Here's how the part is built. I have some questions about the finished solid (model axes, mm). A direction names the side the tool comes from. Coordinates: 2 decimals unless noted, no trailing zeros. Write each loop counter-clockwise with the first axis right and the second up, starting at its lowest first coordinate (ties: lowest second). Pieces come first, ordered by that corner, then holes.
Autodesk Inventor part; units mm, degrees
ref_plane "YZ Plane" through (0, 0, 0) normal (1, 0, 0) x (0, 1, 0)
ref_plane "XZ Plane" through (0, 0, 0) normal (0, 1, 0) x (-1, 0, 0)
ref_plane "XY Plane" through (0, 0, 0) normal (0, 0, 1) x (1, 0, 0)
sketch "Esboço1" plane through (0, 0, 0) normal (0, 1, 0) x (-1, 0, 0)
  line L0 (-20.5, 23.5) -> (20.5, 23.5)
  line L1 (20.5, 23.5) -> (20.5, -23.5)
  line L2 (20.5, -23.5) -> (-20.5, -23.5)
  line L3 (-20.5, -23.5) -> (-20.5, 23.5)
  line L4 (-20.5, 23.5) -> (20.5, -23.5) construction
  line L5 (20.5, 23.5) -> (-20.5, -23.5) construction
  point P0 (0, 0)
  dimension "d0" = 41
  dimension "d1" = 47
extrude "Extrusão1" add sketch "Esboço1" along normal blind 61
shell "Casca1" thickness 2 removed faces 2 at (6.8333, 20.3333, 23.5) at (20.5, 20.3333, -7.8333)
sketch "Esboço4" plane through (-20.5, 0, 23.5) normal (0, 0, 1) x (1, 0, 0)
  line L0 (2, 2) -> (2, 59)
  line L1 (2, 59) -> (15, 59)
  line L2 (15, 59) -> (15, 54.5)
  line L3 (15, 54.5) -> (2, 54.5)
  line L4 (2, 54.5) -> (2, 59)
  line L5 (41, 2) -> (2, 2)
  line L6 (2, 2) -> (15, 2)
  line L7 (15, 2) -> (15, 7.5)
  line L8 (15, 7.5) -> (2, 7.5)
  line L9 (2, 7.5) -> (2, 2)
  arc A0 (7.6282, 59) -> (9.3718, 59) centre (8.5, 57.2) ccw
  circle A1 centre (8.3, 4.5) radius 2
  line L10 (41, 0) -> (0, 0)
  line L11 (0, 0) -> (0, 61)
  line L12 (0, 61) -> (41, 61)
  point P0 (20.5, 0)
  dimension "d15" = 13
  dimension "d16" = 4.5
  dimension "d17" = 13
  dimension "d18" = 5.5
  dimension "d19" = 4
  dimension "d20" = 4
  dimension "d21" = 4.5
  dimension "d22" = 8.3
  dimension "d23" = 3.8
  dimension "d24" = 8.5
extrude "Extrusão2" add sketch "Esboço4" against normal blind 3 contours L0 L1 A0 L2 L3 | L0 L8 L7 L5
fillet "Arredondamento4" radius 4 2 edges at (20.5, 60, 23.5) (20.5, 1, 23.5)
sketch "Esboço11" plane through (-18.5, 2, -21.5) normal (1, 0, 0) x (0, 0, -1)
  line L0 (-42, 5.5) -> (-42, 0)
  line L1 (-45, -2) -> (2, -2)
  line L2 (-42, 5.5) -> (-37.8, 5.5)
  line L3 (-37.8, 5.5) -> (-37.8, -2)
  line L4 (-37.8, -2) -> (-42, -2)
  line L5 (-42, -2) -> (-42, 5.5)
  line L6 (-42, 57) -> (-42, 52.5)
  line L7 (-42, 52.5) -> (-37.8, 52.5)
  line L8 (-37.8, 52.5) -> (-37.8, 59.7447)
  line L9 (-37.8, 59.7447) -> (-42, 59.7447)
  line L10 (-42, 59.7447) -> (-42, 52.5)
  point P0 (-21.5, -2)
  dimension "d47" = 4.2
  dimension "d48" = 4.2
extrude "Extrusão8" cut sketch "Esboço11" along normal blind 13 and the other way blind 2
sketch "Esboço12" plane through (-18.5, 2, -21.5) normal (1, 0, 0) x (0, 0, -1)
  line L0 (-37.8, -2) -> (-37.8, 0)
  line L1 (-37.8, -2) -> (-35.8, -2)
  line L2 (-35.8, -2) -> (-35.8, 8)
  line L3 (-35.8, 8) -> (-37.8, 8)
  line L4 (-37.8, 8) -> (-37.8, -2)
  line L5 (-45, 5.5) -> (-42, 5.5)
  line L6 (-45, 5.5) -> (-37.8, 5.5)
  line L7 (-37.8, 5.5) -> (-37.8, 8)
  line L8 (-37.8, 8) -> (-45, 8)
  line L9 (-45, 8) -> (-45, 5.5)
  line L10 (-45, 52.5) -> (-42, 52.5)
  line L11 (-45, 52.5) -> (-35.8, 52.5)
  line L12 (-35.8, 52.5) -> (-35.8, 50.5)
  line L13 (-35.8, 50.5) -> (-45, 50.5)
  line L14 (-45, 50.5) -> (-45, 52.5)
  line L15 (-37.8, 59) -> (-42, 59)
  line L16 (-35.8, 52.5) -> (-37.8, 52.5)
  line L17 (-37.8, 52.5) -> (-37.8, 59)
  line L18 (-37.8, 59) -> (-35.8, 59)
  line L19 (-35.8, 59) -> (-35.8, 52.5)
  point P0 (-21.5, -2)
  dimension "d53" = 2
  dimension "d54" = 10
  dimension "d55" = 9.2
  dimension "d56" = 2
extrude "Extrusão9" add sketch "Esboço12" along normal blind 13
sketch "Esboço13" plane through (-5.5, 54.5, 16.3) normal (1, 0, 0) x (0, 0, -1)
  line L0 (2, -44.5) -> (-7.2, -44.5)
  line L1 (2, -52.5) -> (2, -44.5)
  line L2 (-7.2, -44.5) -> (2, -44.5)
  line L3 (2, -44.5) -> (2, -52.5)
  line L4 (2, -52.5) -> (-7.2, -52.5)
  line L5 (-7.2, -52.5) -> (-7.2, -44.5)
  line L6 (-7.2, -2) -> (2, -2)
  line L7 (-3.2, 4.5) -> (37.8, 4.5)
  line L8 (-7.2, -2) -> (2, -2)
  line L9 (2, -2) -> (2, 4.5)
  line L10 (2, 4.5) -> (-7.2, 4.5)
  line L11 (-7.2, 4.5) -> (-7.2, -2)
  point P0 (16.3, -54.5)
extrude "Extrusão10" add sketch "Esboço13" along normal blind 2
fillet "Arredondamento5" radius 2 2 edges at (-20.5, 61, 22) (-20.5, 0, 22)
fillet "Arredondamento6" radius 2 2 edges at (-20.5, 61, -3.6) (-20.5, 0, -3.6)
fillet "Arredondamento7" radius 2 5 edges at (-19.9142, 60.4142, -23.5) (1, 61, -23.5) (-19.9142, 0.5858, -23.5) (1, 0, -23.5) (-20.5, 30.5, -23.5)
fillet "Arredondamento10" radius 1 2 edges at (-3.5, 52.5, 18.9) (-3.5, 10, 18.9)
properties part number "Caixa KS"
1. I want a section at B-B (x = -12). State how many separate pieces and enclosed holes the cut face has, then the cut area to 3 significant figures.
2. On a 3-axis mill with a long thin cutter (end or side, diameter ignored), from which of +Z, -Z, +X, -X, +Y, -Y can I reach the whole of each face in a straight line? I mean faces 4 (the face through (1.27, 0.57, -22.9)), 5 (the face through (-13, 58, 16.3)), 6 (the face through (-5.5, 4, 18)), 7 (the face through (-19.9, 0.57, 21.98)), 8 (the face through (-11, 56, 14.3)). Say none if no direction works.
3. For pin 1 Ø12 at (x, y) = (-2.5, 15.5) entering from +Z; pin 2 Ø4 at (x, y) = (-2.5, 39.5) entering from +Z; pin 3 Ø2 at (y, z) = (6, 17.5) entering from +X; pin 4 Ø2 at (y, z) = (2, 17.5) entering from -X, each with a flat end and sliding along its axis, tell me the tip position at first contact or that it passes through.
4. I want a section at A-A (y = 4.5). List the corners of the cut face in (x, z) for me, then the cut area to 3 significant figures.
5. If I drill on line 1 (Y direction, x = -12.2, z = 22.15); line 2 (Y direction, x = -5, z = -3.5); line 3 (Z direction, x = -13.5, y = 51.5), over which ranges is the centre line in solid material (lowest first)?
6. I want a section at D-D (y = 17). List the corners of the cut face in (x, z) for me, then the cut area to 3 significant figures.
7. Thinking about a two-plate mould opening in Y: for faces 1 (the face through (-19.93, 30.1, -22.9)), 2 (the face through (0.73, 60.43, -22.9)), 3 (the face through (-12, 10, 19)), which applies, pulls with the +Y half, pulls with the -Y half, needs draft (parallel to the pull), parting line crosses it, or undercut?
8. I want a section at C-C (z = -6). List the corners of the cut face in (x, y) for me, then the cut area to 3 significant figures.
Response values:
1. separate pieces: 3
1. enclosed holes: 0
1. area: 352 mm2
2. face 4: -Z, +X, -X, -Y
2. face 5: -X, +Y
2. face 6: -X, -Y
2. face 7: +Z, -Z, -X, -Y
2. face 8: +X
3. pin 1: stops at z = 23.5
3. pin 2: stops at z = -21.5
3. pin 3: stops at x = -3.5
3. pin 4: stops at x = -5.5
4. outline: (-20.5, -21.5) arc R2 ccw to (-18.5, -23.5) - (20.5, -23.5) - (20.5, -21.5) - (-18.5, -21.5) - (-18.5, 14.3) - (-3.5, 14.3) - (-3.5, 23.5) - (-10.2, 23.5) - (-10.2, 20.5) - (-5.5, 20.5) - (-5.5, 16.3) - (-20.5, 16.3) - close; (-20.5, 20.5) - (-14.2, 20.5) - (-14.2, 23.5) - (-20.5, 23.5) - close
4. area: 234 mm2
5. line 1: y = 0 to 2.5, 6.5 to 10, 52.5 to 55.21, 59 to 61
5. line 2: y = 0 to 2, 59 to 61
5. line 3: z = -23.5 to -21.5
6. outline: (-20.5, -21.5) arc R2 ccw to (-18.5, -23.5) - (20.5, -23.5) - (20.5, -21.5) - (-18.5, -21.5) - (-18.5, 23.5) - (-20.5, 23.5) - close
6. area: 171 mm2
7. face 1: needs draft
7. face 2: pulls with the +Y half
7. face 3: undercut
8. outline: (-20.5, 2) arc R2 ccw to (-18.5, 0) - (20.5, 0) - (20.5, 2) - (-18.5, 2) - (-18.5, 59) - (20.5, 59) - (20.5, 61) - (-18.5, 61) arc R2 ccw to (-20.5, 59) - close
8. area: 276 mm2
